Can you work these out from the model? Positions are in its coordinate system, mm. Face numbers are marked on the shaded views. A direction names the side the tool comes from. Give positions to 0.01 mm unless a question says otherwise; leave off trailing zeros. Order: outer loops, then holes, each group sorted by start corner. A loop starts at its lowest first (then second) coordinate and runs counter-clockwise, first axis right, second up.
Item 1: I'm going to push flat-ended pins straight in: pin 1 Ø3 at (x, z) = (-1, 24) entering from +Y; pin 2 Ø5 at (x, z) = (-5.5, 9) entering from +Y; pin 3 Ø6 at (x, y) = (-2, 5.5) entering from +Z; pin 4 Ø1.5 at (x, y) = (-6, 1.5) entering from +Z. Where does each tip first touch, or does it pass through?
Item 2: I want a section at D-D, the plane y = 5. Write out the boundary of the cut face in (x, z) (3 decimals).
Item 3: Which directions (+Z, -Z, +X, -X, +Y, -Y) give clear straight access to the entire face, cutting with the end or side of a thin tool? Please do the marked faces 4, 5, 6 and 7.
Item 4: If we mould it in two halves opening along Z, with no side actions, what happens to the marked faces 1, 2 and 3? For each: +Z half, -Z half, draft (parallel to the pull), parting line (faces both ways), or undercut.
Item 5: I want a section at A-A, the plane z = 25. Write out the boundary of the cut face in (x, y) (3 decimals).
Item 6: I want a section at B-B, the plane x = 1. Write out the boundary of the cut face in (y, z).
Item 7: If I drill on line 1 along Z through (x, y) = (4.05, 5); line 2 along Z through (x, y) = (2.75, 2.25); line 3 along Y through (x, z) = (4.45, 25), over which ranges is the centre line in solid material (lowest first)?
Item 8: I want a section at C-C, the plane y = 9.25. Write out the boundary of the cut face in (x, z), then the cut area to 3 significant figures.
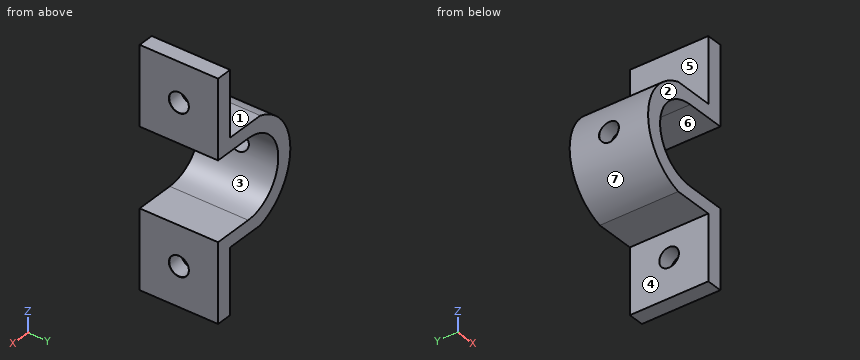
```python
from build123d import *

# Parameters (mm, degrees)
EXTRUDE_1_DEPTH              = 10
HOLE_WIZARD_M3_2_D           = 2.5
HOLE_WIZARD_M3_2_CSINK_D     = 2.55
HOLE_WIZARD_M3_2_CSINK_ANGLE = 90
SKETCH_15_W                  = 10
SKETCH_15_H                  = 10
EXTRUDE_2_DEPTH              = 5
HOLE_WIZARD_M3_1_D           = 2.5
HOLE_WIZARD_M3_1_CSINK_D     = 2.55
HOLE_WIZARD_M3_1_CSINK_ANGLE = 90
SKETCH_21_W                  = 8.291796068
SKETCH_21_H                  = 10
CUT_EXTRUDE_2_DEPTH          = 5


with BuildPart() as part:
    # 草图1 → 凸台-拉伸1 (new body)
    with BuildSketch(Plane(origin=(0, 0, 0), x_dir=(1, 0, 0), z_dir=(0, 1, 0))):
        with BuildLine():
            Line((0, 0), (0, -10))
            ThreePointArc((0, -10), (-5, -15), (0, -20))
            Line((0, -20), (0, -30))
            Line((0, -30), (-2, -30))
            Line((-2, -30), (-2, -21.708203932))
            ThreePointArc((-2, -21.708203932), (-7, -15), (-2, -8.291796068))
            Line((-2, -8.291796068), (-2, 0))
            Line((-2, 0), (0, 0))
        make_face()
    extrude(amount=EXTRUDE_1_DEPTH)

    # M3 螺纹孔的螺纹孔钻头2 (through all)
    with Locations(Plane.ZY.offset(7)):
        with Locations((15, 5)):
            CounterSinkHole(HOLE_WIZARD_M3_2_D / 2, HOLE_WIZARD_M3_2_CSINK_D / 2, counter_sink_angle=HOLE_WIZARD_M3_2_CSINK_ANGLE)

    # 草图15 → 凸台-拉伸2 (add)
    with BuildSketch(Plane(origin=(0, 0, 0), x_dir=(0, 0, -1), z_dir=(1, 0, 0))):
        with Locations((-5, 5)):
            Rectangle(SKETCH_15_W, SKETCH_15_H)
        with Locations((-25, 5)):
            Rectangle(SKETCH_15_W, SKETCH_15_H)
    extrude(amount=EXTRUDE_2_DEPTH)

    # M3 螺纹孔的螺纹孔钻头1 (through all)
    with Locations(Plane(origin=(5, 0, 0), x_dir=(0, 0, -1), z_dir=(1, 0, 0))):
        with Locations((-5, 5), (-25, 5)):
            CounterSinkHole(HOLE_WIZARD_M3_1_D / 2, HOLE_WIZARD_M3_1_CSINK_D / 2, counter_sink_angle=HOLE_WIZARD_M3_1_CSINK_ANGLE)

    # 草图21 → 切除-拉伸2 (cut)
    with BuildSketch(Plane.ZY.offset(2)):
        with Locations((4.145898034, 5)):
            Rectangle(SKETCH_21_W, SKETCH_21_H)
        with Locations((25.854101966, 5)):
            Rectangle(SKETCH_21_W, SKETCH_21_H)
    extrude(amount=-CUT_EXTRUDE_2_DEPTH, mode=Mode.SUBTRACT)


solid = part.part
```
Results list:
1. pin 1: passes through
1. pin 2: stops at y = 10
1. pin 3: stops at z = 21.71
1. pin 4: stops at z = 19.63
2. outline: (-6.887, 13.75) arc R7 ccw to (-2, 8.292) - (3, 8.292) - (3, 6.25) - (4.975, 6.25) - (5, 6.275) - (5, 10) - (0, 10) arc R5 cw to (-4.841, 13.75) - close; (-6.887, 16.25) - (-4.841, 16.25) arc R5 cw to (0, 20) - (5, 20) - (5, 23.725) - (4.975, 23.75) - (3, 23.75) - (3, 21.708) - (-2, 21.708) arc R7 ccw to start; (3, 0) - (5, 0) - (5, 3.725) - (4.975, 3.75) - (3, 3.75) - close; (3, 26.25) - (4.975, 26.25) - (5, 26.275) - (5, 30) - (3, 30) - close
3. face 4: -Z, -X, +Y, -Y
3. face 5: +Z, -X, +Y, -Y
3. face 6: +X, +Y, -Y
3. face 7: -X, +Y, -Y
4. face 1: +Z half
4. face 2: draft
4. face 3: undercut
5. outline: (3, 0) - (5, 0) - (5, 3.725) - (4.975, 3.75) - (3, 3.75) - close; (3, 6.25) - (4.975, 6.25) - (5, 6.275) - (5, 10) - (3, 10) - close
6. outline: (0, 8.29) - (10, 8.29) - (10, 10) - (0, 10) - close; (0, 20) - (10, 20) - (10, 21.71) - (0, 21.71) - close
7. line 1: z = 0 to 3.75, 6.25 to 10, 20 to 23.75, 26.25 to 30
7. line 2: z = 8.29 to 10, 20 to 21.71
7. line 3: y = 0 to 3.75, 6.25 to 10
8. outline: (-2, 8.29) - (3, 8.29) - (3, 0) - (5, 0) - (5, 10) - (0, 10) arc R5 cw to (0, 20) - (5, 20) - (5, 30) - (3, 30) - (3, 21.71) - (-2, 21.71) arc R7 ccw to start
8. area: 87.2 mm2
